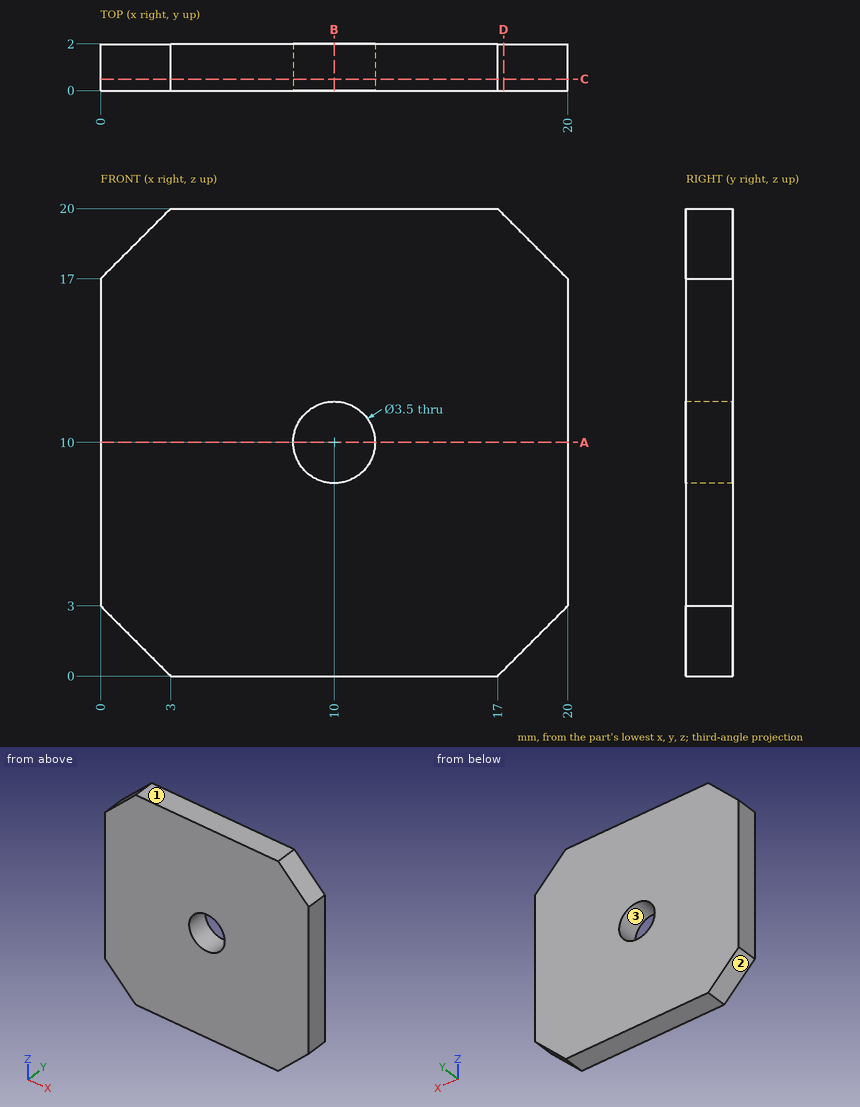
The drawing under review shows one solid part. Ordinate dimensions are in mm from its lowest x, y, z. Coordinates: 2 decimals unless noted, no trailing zeros. Order: outer loops, then holes, each group sorted by start corner. A loop starts at its lowest first (then second) coordinate and runs counter-clockwise, first axis right, second up. Notation, with made-up numbers: M 30.25,66 L 58.25,66 A30 cw 58.25,94 Z; hole C 50.5,84 d4. An arc over 180 degrees is marked long. One line per question, with ' | ' between items.
(1) Add section C-C, the plane y = 0.5. Write out the cut boundary in (x, z).
Geometry results:
outline: M 0,3 L 3,0 L 17,0 L 20,3 L 20,17 L 17,20 L 3,20 L 0,17 Z; hole C 10,10 d3.5
(2) The part is to be moulded in two halves that separate along Z. For the marked faces 1, 2 and 3, say which applies: +Z half, -Z half, draft (parallel to the pull), parting line (faces both ways), or undercut.
Geometry results:
face 1: +Z half | face 2: -Z half | face 3: undercut
(3) Add section A-A, the plane z = 10. Write out the cut boundary in (x, y).
Geometry results:
outline: M 0,0 L 8.25,0 L 8.25,2 L 0,2 Z; M 11.75,0 L 20,0 L 20,2 L 11.75,2 Z
(4) For probe 1 along X at (y, z) = (0.6, 10); probe 2 along X at (y, z) = (1.25, 11); probe 3 along Z at (x, y) = (8.5, 1.1), list the stretches that pass through material, from the lowest coordinate up. Write a range as from..to.
Geometry results:
probe 1: x = 0..8.25, 11.75..20 | probe 2: x = 0..8.56, 11.44..20 | probe 3: z = 0..9.1, 10.9..20
(5) Add section D-D, the plane x = 17.25. Write out the cut boundary in (y, z), then the cut area to 3 significant figures.
Geometry results:
outline: M 0,0.25 L 2,0.25 L 2,19.75 L 0,19.75 Z | area: 39.0 mm²
(6) Add section B-B, the plane x = 10. Write out the cut boundary in (y, z), then the cut area to 3 significant figures.
Geometry results:
outline: M 0,0 L 2,0 L 2,8.25 L 0,8.25 Z; M 0,11.75 L 2,11.75 L 2,20 L 0,20 Z | area: 33.0 mm²
